Build history of the part. All positions in model axes, mm. Coordinates: 2 decimals unless noted, no trailing zeros. Write each loop counter-clockwise with the first axis right and the second up, starting at its lowest first coordinate (ties: lowest second). Pieces come first, ordered by that corner, then holes.
from build123d import *

# Parameters (mm, degrees)
SKETCH1_R               = 25.4
SKETCH1_R_2             = 22.225
BOSS_EXTRUDE1_DEPTH     = 285.115
SKETCH2_R               = 2.4892
CUT_EXTRUDE1_DEPTH      = 26.4
CUT_EXTRUDE1_DEPTH_BACK = 26.4
SKETCH3_R               = 2.4892
CUT_EXTRUDE2_DEPTH      = 26.4000001
CUT_EXTRUDE2_DEPTH_BACK = 26.4000001


with BuildPart() as part:
    # Sketch1 → Boss-Extrude1 (new body, symmetric)
    with BuildSketch(Plane(origin=(0, 0, 0), x_dir=(0, 0, -1), z_dir=(1, 0, 0))):
        Circle(SKETCH1_R)
        Circle(SKETCH1_R_2, mode=Mode.SUBTRACT)
    extrude(amount=BOSS_EXTRUDE1_DEPTH, both=True)

    # Sketch2 → Cut-Extrude1 (cut, two sides)
    with BuildSketch(Plane.XY) as cut_extrude1_sk:
        with Locations((-275.59, 0)):
            Circle(SKETCH2_R)
        with Locations((275.59, 0)):
            Circle(SKETCH2_R)
    extrude(amount=CUT_EXTRUDE1_DEPTH, mode=Mode.SUBTRACT)
    extrude(cut_extrude1_sk.sketch, amount=-CUT_EXTRUDE1_DEPTH_BACK, mode=Mode.SUBTRACT)

    # Sketch3 → Cut-Extrude2 (cut, two sides)
    with BuildSketch(Plane(origin=(0, 0, 0), x_dir=(1, 0, 0), z_dir=(0, 1, 0))) as cut_extrude2_sk:
        with Locations((-275.59, 0)):
            Circle(SKETCH3_R)
        with Locations((275.59, 0)):
            Circle(SKETCH3_R)
    extrude(amount=CUT_EXTRUDE2_DEPTH, mode=Mode.SUBTRACT)
    extrude(cut_extrude2_sk.sketch, amount=-CUT_EXTRUDE2_DEPTH_BACK, mode=Mode.SUBTRACT)


solid = part.part
(1) Two-plate mould, pull along Y, no slides. Class faces 1 (the flat face through (285.115, -22.5, 0.1)), 2 (the cylindrical face through (3.992, -24.796, 5.506)), 3 (the cylindrical face through (-3.992, 6.676, -21.199)): pulls with the +Y half, pulls with the -Y half, needs draft (parallel to the pull), parting line crosses it, or undercut.
(2) Slice it at A-A, the plane z = 13. List the corners of the cut face in (x, y) (3 decimals), and give its area (3 significant figures).
(3) Slice it at C-C, the plane z = -16. List the corners of the cut face in (x, y) (3 decimals).
(4) Flat gauge pins, fed straight in: P1, Ø3, axis at x = 275.59, z = 0, coming from the +Y side; P2, Ø5.5, axis at x = 275.59, z = 0, coming from the +Y side; P3, Ø1, axis at x = 204, y = 18.5, coming from the -Z side; P4, Ø1.5, axis at x = -10.5, z = -10, coming from the -Y side. Where does each tip first touch, or does it go through?
(5) Slice it at B-B, the plane x = -51. List the corners of the cut face in (y, z) (3 decimals), and give its area (3 significant figures).
(6) Probe L1, parallel to X at y = 24, z = 0 (3 decimals); L2, parallel to Z at x = -132, y = -2; L3, parallel to Y at x = 52, z = -1. List the from-to ranges inside material, lowest first.
Results:
1. face 1: needs draft
1. face 2: parting line crosses it
1. face 3: undercut
2. outline: (-285.115, -21.821) - (285.115, -21.821) - (285.115, -18.026) - (-285.115, -18.026) - close; (-285.115, 18.026) - (285.115, 18.026) - (285.115, 21.821) - (-285.115, 21.821) - close
2. area: 4,330 mm2
3. outline: (-285.115, -19.727) - (285.115, -19.727) - (285.115, -15.426) - (-285.115, -15.426) - close; (-285.115, 15.426) - (285.115, 15.426) - (285.115, 19.727) - (-285.115, 19.727) - close
4. P1: passes through
4. P2: stops at y = 25.4
4. P3: stops at z = -17.92
4. P4: stops at y = -23.66
5. outline: circle Ø50.8 at (0, 0); hole circle Ø44.45 at (0, 0)
5. area: 475 mm2
6. L1: x = -285.115 to -278.079, -273.101 to 273.101, 278.079 to 285.115
6. L2: z = -25.32 to -22.13, 22.13 to 25.32
6. L3: y = -25.38 to -22.2, 22.2 to 25.38
